from build123d import *

# Parameters (mm, degrees)
SKETCH1_W           = 45
SKETCH1_H           = 45
SKETCH1_R           = 1.8
BOSS_EXTRUDE1_DEPTH = 0.8
SKETCH2_W           = 2.26484959
SKETCH2_H           = 1
SKETCH2_W_2         = 2.264849589
BOSS_EXTRUDE2_DEPTH = 1.6
SKETCH3_W           = 20.5
SKETCH3_H           = 36
SPARK_CORE_DEPTH    = 14.7


with BuildPart() as part:
    # Sketch1 → Boss-Extrude1 (new, symmetric)
    with BuildSketch(Plane(origin=(0, 0, 0), x_dir=(1, 0, 0), z_dir=(0, 1, 0))):
        Rectangle(SKETCH1_W, SKETCH1_H)
        with Locations(Location((-17.65, 17.65, 0), (0, 0, 270))):
            Circle(SKETCH1_R, mode=Mode.SUBTRACT)
        with Locations(Location((17.65, 17.65, 0), (0, 0, 270))):
            Circle(SKETCH1_R, mode=Mode.SUBTRACT)
        with Locations(Location((17.65, -17.65, 0), (0, 0, 270))):
            Circle(SKETCH1_R, mode=Mode.SUBTRACT)
        with Locations(Location((-17.65, -17.65, 0), (0, 0, 270))):
            Circle(SKETCH1_R, mode=Mode.SUBTRACT)
    extrude(amount=BOSS_EXTRUDE1_DEPTH, both=True)

    # Sketch2 → Boss-Extrude2 (add)
    with BuildSketch(Plane(origin=(0, 0.8, 0), x_dir=(1, 0, 0), z_dir=(0, 1, 0))):
        with Locations((-16.569776824, 23)):
            Rectangle(SKETCH2_W, SKETCH2_H)
        with Locations((-13.030949341, 23)):
            Rectangle(SKETCH2_W_2, SKETCH2_H)
        with Locations((-8.288920513, 23)):
            Rectangle(SKETCH2_W, SKETCH2_H)
        with Locations((-4.113104082, 23)):
            Rectangle(SKETCH2_W_2, SKETCH2_H)
        with Locations((7.140367316, 23)):
            Rectangle(SKETCH2_W_2, SKETCH2_H)
        with Locations((12.059337518, 23)):
            Rectangle(SKETCH2_W_2, SKETCH2_H)
        with Locations((16.412095322, 23)):
            Rectangle(SKETCH2_W, SKETCH2_H)
    extrude(amount=-BOSS_EXTRUDE2_DEPTH)

    # Sketch3 → Spark Core (add)
    with BuildSketch(Plane(origin=(0, 0.8, 0), x_dir=(1, 0, 0), z_dir=(0, 1, 0))):
        with Locations((3.61, 0.1)):
            Rectangle(SKETCH3_W, SKETCH3_H)
    extrude(amount=SPARK_CORE_DEPTH)


solid = part.part
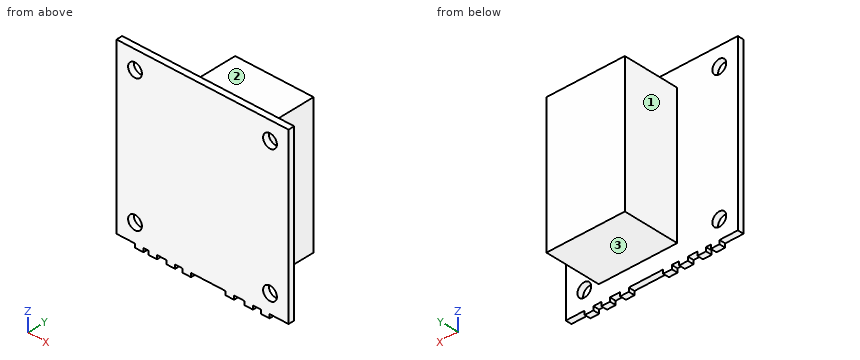
Could you check a few things on this model? Use its own coordinates, in mm. Face numbers are marked on the shaded views. A direction names the side the tool comes from. Give positions to 0.01 mm unless a question says otherwise; leave off trailing zeros. Write each loop counter-clockwise with the first axis right and the second up, starting at its lowest first coordinate (ties: lowest second). Pieces come first, ordered by that corner, then holes. Notation, with made-up numbers: (73, 68.25) - (83, 68.25) arc R24 ccw to (83, 78.25) - close; hole circle Ø11 at (-0.75, -5.75). An arc over 180 degrees is marked (long way). Use CSV: the item, a comma, the result in double quotes. Start each with the question number.
Item 1: I'm going to push flat-ended pins straight in: pin 1 (6 mm diameter, centred on x = -3, y = 6, fed in from +Z); pin 2 (6 mm diameter, centred on y = 8, z = -5, fed in from +X); pin 3 (0.8 mm diameter, centred on y = 0, z = -23, fed in from -X). Where does each tip first touch, or does it pass through?
Item 2: I want a section at C-C, the plane y = 13.5. Please give me the cut outline in (x, z).
Item 3: I want a section at D-D, the plane x = -8. Please give me the cut outline in (y, z), then the cut area to 3 significant figures.
Item 4: I want a section at B-B, the plane x = 1. Please give me the cut outline in (y, z).
Item 5: For the marked faces 1, 2 and 3, which set-ups out of +Z, -Z, +X, -X, +Y, -Y let a thin tool reach every point of the face, with its end or its side?
Item 6: I want a section at A-A, the plane z = -2.5. Please give me the cut outline in (x, y), then the cut area to 3 significant figures.
Item 7: If I drill on line 1 along X through (y, z) = (-0.1, 17.65); line 2 along X through (y, z) = (7.75, 14); line 3 along Y through (x, z) = (-10, 6), over which ranges is the centre line in solid material (lowest first)?
Findings:
1,pin 1,"stops at z = 17.9"
1,pin 2,"stops at x = 13.86"
1,pin 3,"stops at x = -17.7"
2,outline,"(-6.64, -18.1) - (13.86, -18.1) - (13.86, 17.9) - (-6.64, 17.9) - close"
3,outline,"(-0.8, -23.5) - (0.8, -23.5) - (0.8, 22.5) - (-0.8, 22.5) - close"
3,area,"73.6 mm2"
4,outline,"(-0.8, -22.5) - (0.8, -22.5) - (0.8, -18.1) - (15.5, -18.1) - (15.5, 17.9) - (0.8, 17.9) - (0.8, 22.5) - (-0.8, 22.5) - close"
5,face 1,"+Z, -Z, -X, +Y"
5,face 2,"+Z, +X, -X, +Y"
5,face 3,"-Z, +X, -X, +Y"
6,outline,"(-22.5, -0.8) - (22.5, -0.8) - (22.5, 0.8) - (13.86, 0.8) - (13.86, 15.5) - (-6.64, 15.5) - (-6.64, 0.8) - (-22.5, 0.8) - close"
6,area,"373 mm2"
7,line 1,"x = -22.5 to -19.45, -15.85 to 15.85, 19.45 to 22.5"
7,line 2,"x = -6.64 to 13.86"
7,line 3,"y = -0.8 to 0.8"
